```python
from build123d import *

# Parameters (mm, degrees)
SKETCH1_W                = 120
SKETCH1_H                = 50
BOSS_EXTRUDE1_DEPTH      = 8
SKETCH2_W                = 8
SKETCH2_H                = 40
BOSS_EXTRUDE2_DEPTH      = 37
FILLET1_R                = 20
BOSS_EXTRUDE3_DEPTH      = 10
BOSS_EXTRUDE3_DEPTH_BACK = 120
SKETCH3_R                = 4
FILLET2_R                = 2


with BuildPart() as part:
    # Sketch1 → Boss-Extrude1 (new body)
    with BuildSketch(Plane(origin=(0, 0, 0), x_dir=(1, 0, 0), z_dir=(0, 1, 0))):
        Rectangle(SKETCH1_W, SKETCH1_H)
    extrude(amount=BOSS_EXTRUDE1_DEPTH)

    # Sketch2 → Boss-Extrude2 (add)
    with BuildSketch(Plane(origin=(0, 8, 0), x_dir=(1, 0, 0), z_dir=(0, 1, 0))):
        with Locations((-51, 0)):
            Rectangle(SKETCH2_W, SKETCH2_H)
        with Locations((51, 0)):
            Rectangle(SKETCH2_W, SKETCH2_H)
    extrude(amount=BOSS_EXTRUDE2_DEPTH)

    # Fillet1
    fillet1_edges = [part.edges().sort_by_distance(p)[0] for p in [
        (51, 45, -20),
        (51, 45, 20),
        (-51, 45, -20),
        (-51, 45, 20),
    ]]
    fillet(fillet1_edges, radius=FILLET1_R - 0.0001)  # a hair under: the kernel refuses the full size

    # Sketch3 → Boss-Extrude3 (add, two sides: drawn at the far end of the back side and taken through both)
    with BuildSketch(Plane.ZY.offset(55).offset(-BOSS_EXTRUDE3_DEPTH_BACK)):
        with Locations((0, 30)):
            Circle(SKETCH3_R)
    extrude(amount=BOSS_EXTRUDE3_DEPTH + BOSS_EXTRUDE3_DEPTH_BACK)

    # Fillet2
    fillet2_edges = [part.edges().sort_by_distance(p)[0] for p in [
        (-60, 4, -25),
        (60, 4, -25),
        (60, 4, 25),
        (-60, 4, 25),
    ]]
    fillet(fillet2_edges, radius=FILLET2_R)


solid = part.part
```
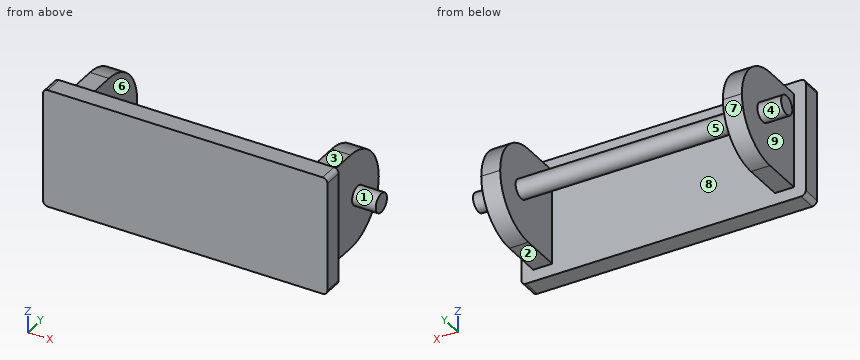
For this review, take the finished solid that the model builds, in its own axes (mm). Face numbers are marked on the shaded views. A direction names the side the tool comes from. Give positions to 0.01 mm unless a question says otherwise; leave off trailing zeros. Loops run counter-clockwise (first coordinate to the right, second up) from the corner with the lowest first, then second, coordinate; pieces in that order, holes last. Notation, with made-up numbers: M 24,36 L 71,36 A20 ccw 71,61 Z; hole C -37,81 d2. An arc over 180 degrees is marked long. One line per item, written item: value. Start each with the question number.
Q1. Add section C-C (x = -13). Give the boundary of the cut face in (y, z).
Q2. Add section B-B (y = 5). Give the boundary of the cut face in (x, z).
Q3. Add section A-A (y = 21.5). Give the boundary of the cut face in (x, z).
Q4. Clearance check with flat-ended pins moving along their axes: pin 1 Ø12 at (y, z) = (28, 11) entering from -X; pin 2 Ø15 at (x, z) = (16, 4) entering from +Y; pin 3 Ø1 at (x, y) = (-50, 27.5) entering from -Z. State where each tip first meets the part, or that it passes through.
Q5. Draft analysis for pull direction X (two halves, no side actions). For the marked faces 6, 7, 8 and 9, state which applies: released by +X, released by -X, zero draft, split by the parting line, or undercut.
Q6. Machinability: for the marked faces 1, 2, 3, 4 and 5, which of the approach directions +Z, -Z, +X, -X, +Y, -Y give a long, thin tool a straight path to every point of the face, cutting with its end or side? Answer none if there is none.
Q7. For L1, parallel to X at y = 27, z = 3; L2, parallel to Y at x = 49.5, z = -1; L3, parallel to Y at x = 20, z = -7.5, list the stretches that pass through material, from the lowest coordinate up.
Reply:
1. outline: M 0,-25 L 8,-25 L 8,25 L 0,25 Z; C 30,0 d8
2. outline: M -60,-23 A2 ccw -58,-25 L 58,-25 A2 ccw 60,-23 L 60,23 A2 ccw 58,25 L -58,25 A2 ccw -60,23 Z
3. outline: M -55,-20 L -47,-20 L -47,20 L -55,20 Z; M 47,-20 L 55,-20 L 55,20 L 47,20 Z
4. pin 1: x = -55
4. pin 2: y = 34
4. pin 3: z = -19.9
5. face 6: undercut
5. face 7: zero draft
5. face 8: undercut
5. face 9: released by -X
6. face 1: +X
6. face 2: -Z, +X, -X, +Y
6. face 3: +Z, +X, -X, +Y
6. face 4: -X
6. face 5: none
7. L1: -55 to -47, 47 to 55
7. L2: 0 to 44.97
7. L3: 0 to 8
